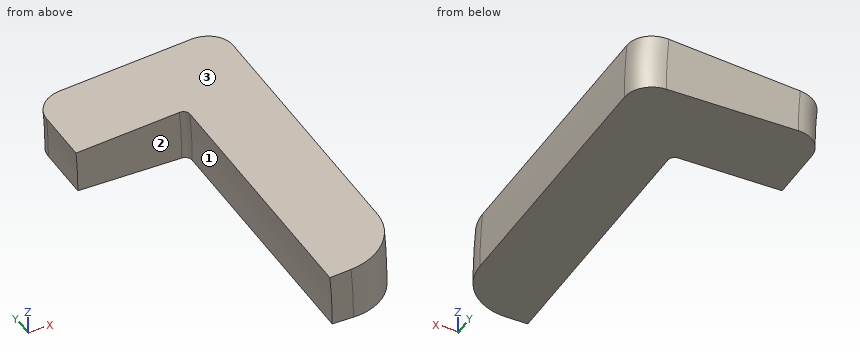
from build123d import *

# Parameters (mm, degrees)
REVOLVE1_ANGLE = 5


with BuildPart() as part:
    # Sketch1 → Revolve1 (revolve)
    with BuildSketch(Plane.XY):
        with BuildLine():
            Line((0, 0), (0, 13.5))
            ThreePointArc((0, 13.5), (-0.146446609, 13.853553391), (-0.5, 14))
            Line((-0.5, 14), (-8, 14))
            Line((-8, 14), (-8, 18.109583933))
            ThreePointArc((-8, 18.109583933), (-7.414213562, 19.523797495), (-6, 20.109583933))
            Line((-6, 20.109583933), (3.533069031, 20.109583933))
            ThreePointArc((3.533069031, 20.109583933), (4.947282593, 19.523797495), (5.533069031, 18.109583933))
            Line((5.533069031, 18.109583933), (5.533069031, 14))
            Line((5.533069031, 14), (5.533069031, 0))
            Line((5.533069031, 0), (5.533069031, -2))
            ThreePointArc((5.533069031, -2), (4.361496156, -4.828427125), (1.533069031, -6))
            Line((1.533069031, -6), (0, -6))
            Line((0, -6), (0, 0))
        make_face()
    revolve(axis=Axis((-43.4, 20.109583933, 0), (0, -1, 0)), revolution_arc=REVOLVE1_ANGLE)


solid = part.part
Read the model definition and answer for the solid it produces. Units are mm, in the model's axes. Face numbers are marked on the shaded views. A direction names the side the tool comes from. Coordinates: 2 decimals unless noted, no trailing zeros. Order: outer loops, then holes, each group sorted by start corner. A loop starts at its lowest first (then second) coordinate and runs counter-clockwise, first axis right, second up. Notation, with made-up numbers: (12, -19) -> (29, -19) arc R19 ccw to (29, -11) -> close; hole circle Ø4 at (20, 2). An arc over 180 degrees is marked (long way). Answer as a JSON object with one key per item and string values.
1) A cutting plane is placed at A-A, the plane y = 14.75. Determine the outline of the cut face in (x, z), plus the area to 3 significant figures.
Model answer:
{"outline": "(-8.13, 3.09) arc R35.4 cw to (-8, 0) -> (5.53, 0) arc R48.93 ccw to (5.35, 4.26) -> close", "area": "49.8 mm²"}
2) Each of these flat-tipped pins is pushed along its axis until it touches: pin 1 (2 mm diameter, centred on x = 3, z = 0.5, fed in from -Y); pin 2 (2 mm diameter, centred on y = 16, z = 1.5, fed in from +X); pin 3 (1.1 mm diameter, centred on x = -3.5, z = 2, fed in from -Y). Where does it stop, or does it pass through?
Model answer:
{"pin 1": "stops at y = -5.97", "pin 2": "stops at x = 5.53", "pin 3": "stops at y = 14"}
3) A cutting plane is placed at B-B, the plane x = 1. Determine the outline of the cut face in (y, z).
Model answer:
{"outline": "(-6, 0) -> (20.11, 0) -> (20.11, 3.88) -> (-6, 3.88) -> close"}
4) Consider line 1 along Y through (x, z) = (-3.5, 1.8); line 2 along X through (y, z) = (8.75, 0.6); line 3 along Z through (x, y) = (-0.5, 16). Determine where each line is inside the solid, lowest interval first. Write a range as from..to.
Model answer:
{"line 1": "y = 14..20.11", "line 2": "x = 0..5.53", "line 3": "z = 0..3.75"}
5) A tool of negligible diameter and unlimited length cuts with its end or side. For the marked faces 1, 2 and 3, from which of +Z, -Z, +X, -X, +Y, -Y can it reach the whole face along a straight path? Write none if from no direction.
Model answer:
{"face 1": "-Z, -X, -Y", "face 2": "+Z, -Z, -X, -Y", "face 3": "+Z, -X, +Y, -Y"}
